from build123d import *

# Parameters (mm, degrees)
SKETCH2_W           = 1
SKETCH2_H           = 35.9
BASE_EXTRUDE_DEPTH  = 11.5
SKETCH3_W           = 11.5
SKETCH3_H           = 25.678293072
BOSS_EXTRUDE1_DEPTH = 7.15
SKETCH4_W           = 5.5
SKETCH4_H           = 19.678293072
CUT_EXTRUDE1_DEPTH  = 5.15
SKETCH5_W           = 5.5
SKETCH5_H           = 7
BOSS_EXTRUDE3_DEPTH = 14.15


with BuildPart() as part:
    # Sketch2 → Base-Extrude (new body)
    with BuildSketch(Plane.XY):
        with Locations((-7.742570808, 38.78)):
            Rectangle(SKETCH2_W, SKETCH2_H)
    extrude(amount=BASE_EXTRUDE_DEPTH)

    # Sketch3 → Boss-Extrude1 (add)
    with BuildSketch(Plane.ZY.offset(8.242570808)):
        with Locations((5.75, 38.78)):
            Rectangle(SKETCH3_W, SKETCH3_H)
    extrude(amount=BOSS_EXTRUDE1_DEPTH)

    # Sketch4 → Cut-Extrude1 (cut)
    with BuildSketch(Plane(origin=(-7.242570808, 0, 0), x_dir=(0, 0, -1), z_dir=(1, 0, 0))):
        with Locations((-5.75, 38.78)):
            Rectangle(SKETCH4_W, SKETCH4_H)
    extrude(amount=-CUT_EXTRUDE1_DEPTH, mode=Mode.SUBTRACT)

    # Sketch5 → Boss-Extrude3 (add)
    with BuildSketch(Plane(origin=(-12.392570808, 0, 0), x_dir=(0, 0, -1), z_dir=(1, 0, 0))):
        with Locations((-5.75, 38.779386514)):
            Rectangle(SKETCH5_W, SKETCH5_H)
    extrude(amount=BOSS_EXTRUDE3_DEPTH)


solid = part.part
The model under review builds one solid part; all positions refer to its coordinate system, in mm. A direction names the side the tool comes from. Give positions to 0.01 mm unless a question says otherwise; leave off trailing zeros. Loops run counter-clockwise (first coordinate to the right, second up) from the corner with the lowest first, then second, coordinate; pieces in that order, holes last. Notation, with made-up numbers: (88, 64.25) -> (113, 64.25) arc R6 cw to (113, 72.25) -> close; hole circle Ø5 at (68.5, 51.5). An arc over 180 degrees is marked (long way). Answer as a JSON object with one key per item and string values. Group by question number.
Q1. Take a section at B-B (y = 44). Write out the cut boundary in (x, z).
Q2. Insertion check: pin 1 (1 mm diameter, centred on x = -10.5, y = 35.5, fed in from -Z); pin 2 (2 mm diameter, centred on x = -11, z = 5.5, fed in from -Y); pin 3 (2 mm diameter, centred on x = -2, y = 37.5, fed in from -Z); pin 4 (1.5 mm diameter, centred on y = 55, z = 5.5, fed in from -X). Each pin has a flat end and moves straight along its axis. Give the tip position at first contact, or say it passes through.
Q3. Tool access review of faces 1 (the flat face through (-3, 39, 8.5)), 2 (the flat face through (-10, 45, 8.5)), 3 (the flat face through (1.757, 39, 6)), 4 (the flat face through (-12, 25.941, 6)), 5 (the flat face through (-8.243, 54, 6)): name each direction out of +Z, -Z, +X, -X, +Y, -Y from which nothing blocks a thin tool from reaching the whole face with its end or side.
Q4. Take a section at D-D (z = 4.25). Write out the cut boundary in (x, y), plus the area to 3 significant figures.
Q5. Take a section at C-C (x = -9). Write out the cut boundary in (y, z), plus the area to 3 significant figures.
Q6. Wall thickness on line 1 along Y through (x, z) = (-9, 2); line 2 along Z through (x, y) = (-1.75, 41); line 3 along X through (y, z) = (38, 9): over which ranges is each line inside the solid? List them lowest first.
Q7. Take a section at A-A (z = 9.5). Write out the cut boundary in (x, y), plus the area to 4 significant figures.
Q8. Draft analysis for pull direction Z (two halves, no side actions). For faces 6 (the flat face through (-3, 39, 3)), 7 (the flat face through (-10, 48.619, 6)), 8 (the flat face through (-8.243, 23, 6)), state which applies: pulls with the +Z half, pulls with the -Z half, needs draft (parallel to the pull), parting line crosses it, or undercut.
Answer below:
{
 "1": {"outline": "(-15.39, 0) -> (-7.24, 0) -> (-7.24, 3) -> (-12.39, 3) -> (-12.39, 8.5) -> (-7.24, 8.5) -> (-7.24, 11.5) -> (-15.39, 11.5) -> close"},
 "2": {"pin 1": "stops at z = 0", "pin 2": "stops at y = 25.94", "pin 3": "stops at z = 3", "pin 4": "stops at x = -8.24"},
 "3": {"face 1": "+Z, +X, +Y, -Y", "face 2": "+X", "face 3": "+Z, -Z, +X, +Y, -Y", "face 4": "+Z, -Z, -X, -Y", "face 5": "+Z, -Z, -X, +Y"},
 "4": {"outline": "(-15.39, 25.94) -> (-8.24, 25.94) -> (-8.24, 20.83) -> (-7.24, 20.83) -> (-7.24, 28.94) -> (-12.39, 28.94) -> (-12.39, 35.28) -> (1.76, 35.28) -> (1.76, 42.28) -> (-12.39, 42.28) -> (-12.39, 48.62) -> (-7.24, 48.62) -> (-7.24, 56.73) -> (-8.24, 56.73) -> (-8.24, 51.62) -> (-15.39, 51.62) -> close", "area": "217 mm2"},
 "5": {"outline": "(25.94, 0) -> (51.62, 0) -> (51.62, 11.5) -> (25.94, 11.5) -> close; hole (28.94, 3) -> (35.28, 3) -> (35.28, 8.5) -> (28.94, 8.5) -> close; hole (42.28, 3) -> (48.62, 3) -> (48.62, 8.5) -> (42.28, 8.5) -> close", "area": "226 mm2"},
 "6": {"line 1": "y = 25.94 to 51.62", "line 2": "z = 3 to 8.5", "line 3": "x = -15.39 to -7.24"},
 "7": {"outline": "(-15.39, 25.94) -> (-8.24, 25.94) -> (-8.24, 20.83) -> (-7.24, 20.83) -> (-7.24, 56.73) -> (-8.24, 56.73) -> (-8.24, 51.62) -> (-15.39, 51.62) -> close", "area": "219.5 mm2"},
 "8": {"face 6": "pulls with the -Z half", "face 7": "undercut", "face 8": "needs draft"}
}
